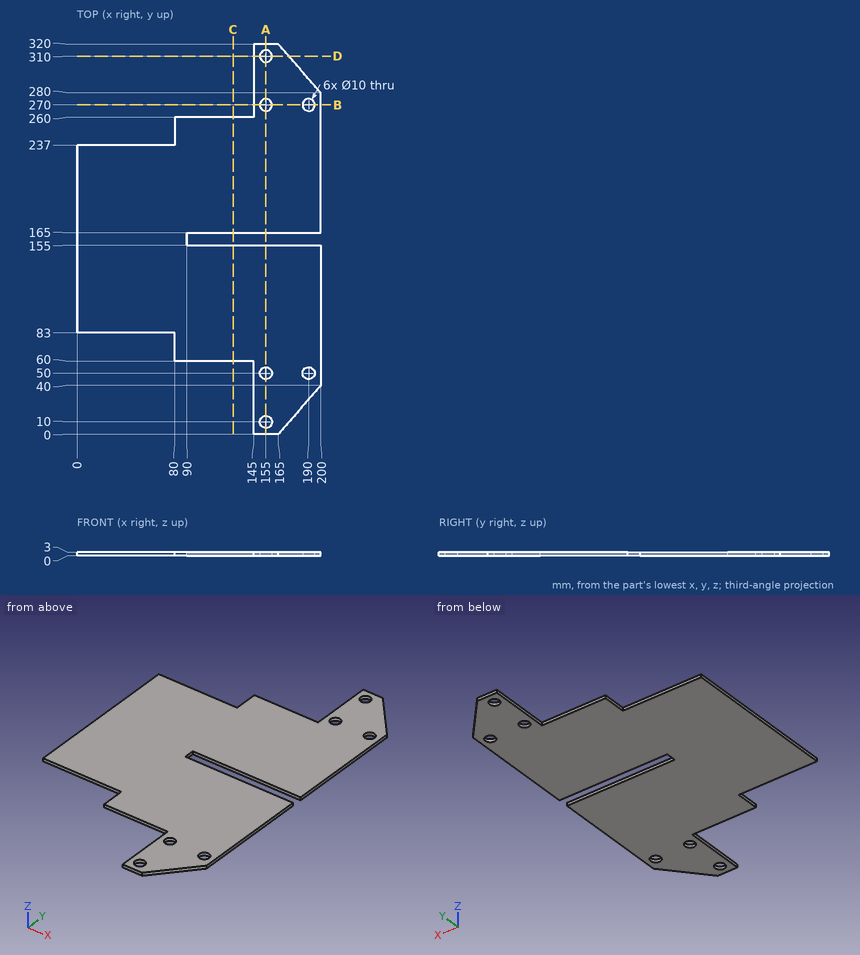
Geometry check sheet. Reference: drawing and pictorial views, mm from the part's lowest x, y, z. Give positions to 0.01 mm unless a question says otherwise; leave off trailing zeros. Order: outer loops, then holes, each group sorted by start corner. A loop starts at its lowest first (then second) coordinate and runs counter-clockwise, first axis right, second up. Notation, with made-up numbers: M 63.25,36 L 95.25,36 A23 cw 95.25,71 Z; hole C 74.25,65.5 d5. An arc over 180 degrees is marked long. Return JSON: item names as keys, results as strings. Group by question number.
1) Scan lines: line 1 (Y direction, x = 155, z = 1.5); line 2 (Y direction, x = 91.5, z = 0.5); line 3 (Y direction, x = 190, z = 2.15). Record each from-to range of solid material in increasing order.
2) Section check A-A on x = 155. Record the cut outline in (y, z).
3) Section check B-B on y = 270. Record the cut outline in (x, z).
4) Go/stop test with flat-tipped pins: pin 1 Ø1 at (y, z) = (204, 1.5) entering from -X; pin 2 Ø0.9 at (y, z) = (246, 1) entering from -X; pin 3 Ø0.9 at (y, z) = (17, 1) entering from -X; pin 4 Ø0.9 at (x, z) = (106, 1) entering from +Y. Record where each tip stops, or that it passes through.
5) Section check C-C on x = 128. Record the cut outline in (y, z).
6) Section check D-D on y = 310. Record the cut outline in (x, z).
Answer block:
{
 "1": {"line 1": "y = 0 to 5, 15 to 45, 55 to 155, 165 to 265, 275 to 305, 315 to 320", "line 2": "y = 60 to 155, 165 to 260", "line 3": "y = 28.57 to 45, 55 to 155, 165 to 265, 275 to 291.43"},
 "2": {"outline": "M 0,0 L 5,0 L 5,3 L 0,3 Z; M 15,0 L 45,0 L 45,3 L 15,3 Z; M 55,0 L 155,0 L 155,3 L 55,3 Z; M 165,0 L 265,0 L 265,3 L 165,3 Z; M 275,0 L 305,0 L 305,3 L 275,3 Z; M 315,0 L 320,0 L 320,3 L 315,3 Z"},
 "3": {"outline": "M 145,0 L 150,0 L 150,3 L 145,3 Z; M 160,0 L 185,0 L 185,3 L 160,3 Z; M 195,0 L 200,0 L 200,3 L 195,3 Z"},
 "4": {"pin 1": "stops at x = 0", "pin 2": "stops at x = 80", "pin 3": "stops at x = 145", "pin 4": "stops at y = 260"},
 "5": {"outline": "M 60,0 L 155,0 L 155,3 L 60,3 Z; M 165,0 L 260,0 L 260,3 L 165,3 Z"},
 "6": {"outline": "M 145,0 L 150,0 L 150,3 L 145,3 Z; M 160,0 L 173.75,0 L 173.75,3 L 160,3 Z"}
}
